from build123d import *

# Parameters (mm, degrees)
SKETCH_1_W          = 100
SKETCH_1_H          = 100
EXTRUDE_1_DEPTH     = 4
SKETCH_4_W          = 100
SKETCH_4_H          = 100
CUT_EXTRUDE_1_DEPTH = 71.823724839
SKETCH_5_R          = 5.9
EXTRUDE_2_DEPTH     = 1
SKETCH_6_R          = 1.5
SKETCH_6_R_2        = 1
CUT_EXTRUDE_2_DEPTH = 43.699531613
SKETCH_7_R          = 2.5
CUT_EXTRUDE_3_DEPTH = 2


with BuildPart() as part:
    # Эскиз1 → Бобышка-Вытянуть1 (new body)
    with BuildSketch(Plane(origin=(0, 0, 0), x_dir=(1, 0, 0), z_dir=(0, 1, 0))):
        Rectangle(SKETCH_1_W, SKETCH_1_H)
    extrude(amount=EXTRUDE_1_DEPTH)

    # Эскиз4 → Вырез-Вытянуть1 (cut, through all)
    with BuildSketch(Plane(origin=(0, 4, 0), x_dir=(1, 0, 0), z_dir=(0, 1, 0))):
        Rectangle(SKETCH_4_W, SKETCH_4_H)
        with BuildLine():
            Line((3.546261356, 21.75), (5.566987298, 25.25))
            ThreePointArc((5.566987298, 25.25), (5.566987298, 25.75), (5.133974596, 26))
            Line((5.133974596, 26), (-5.133974596, 26))
            ThreePointArc((-5.133974596, 26), (-5.566987298, 25.75), (-5.566987298, 25.25))
            Line((-5.566987298, 25.25), (-3.546261356, 21.75))
            ThreePointArc((-3.546261356, 21.75), (-3.546261356, 21.25), (-3.979274058, 21))
            Line((-3.979274058, 21), (-13, 21))
            ThreePointArc((-13, 21), (-17.862198755, 19.352875197), (-20.722235468, 15.089755817))
            ThreePointArc((-20.722235468, 15.089755817), (-23.196926567, 10.739563503), (-27.469608288, 8.133328648))
            ThreePointArc((-27.469608288, 8.133328648), (-33.5, 0), (-27.469608288, -8.133328648))
            ThreePointArc((-27.469608288, -8.133328648), (-23.196926567, -10.739563503), (-20.722235468, -15.089755817))
            ThreePointArc((-20.722235468, -15.089755817), (-17.862198755, -19.352875197), (-13, -21))
            Line((-13, -21), (13, -21))
            ThreePointArc((13, -21), (17.862198755, -19.352875197), (20.722235468, -15.089755817))
            ThreePointArc((20.722235468, -15.089755817), (23.196926567, -10.739563503), (27.469608288, -8.133328648))
            ThreePointArc((27.469608288, -8.133328648), (33.5, 0), (27.469608288, 8.133328648))
            ThreePointArc((27.469608288, 8.133328648), (23.196926567, 10.739563503), (20.722235468, 15.089755817))
            ThreePointArc((20.722235468, 15.089755817), (17.862198755, 19.352875197), (13, 21))
            Line((13, 21), (3.979274058, 21))
            ThreePointArc((3.979274058, 21), (3.546261356, 21.25), (3.546261356, 21.75))
        make_face(mode=Mode.SUBTRACT)
    extrude(amount=-CUT_EXTRUDE_1_DEPTH, mode=Mode.SUBTRACT)

    # Эскиз5 → Бобышка-Вытянуть2 (add)
    with BuildSketch(Plane.XZ):
        with Locations(Location((25, 0, 0), (0, 0, 270))):
            Circle(SKETCH_5_R)
        with Locations(Location((-25, 0, 0), (0, 0, 270))):
            Circle(SKETCH_5_R)
        with BuildLine():
            Line((-0.970460198, 14.023475383), (0.970460198, 14.023475383))
            ThreePointArc((0.970460198, 14.023475383), (1.700884179, 14.199930228), (2.270199596, 14.690374372))
            ThreePointArc((2.270199596, 14.690374372), (15.793250353, 15.793250353), (14.690374372, 2.270199596))
            ThreePointArc((14.690374372, 2.270199596), (14.199930228, 1.700884179), (14.023475383, 0.970460198))
            Line((14.023475383, 0.970460198), (14.023475383, -0.970460198))
            ThreePointArc((14.023475383, -0.970460198), (14.199930228, -1.700884179), (14.690374372, -2.270199596))
            ThreePointArc((14.690374372, -2.270199596), (15.793250353, -15.793250353), (2.270199596, -14.690374372))
            ThreePointArc((2.270199596, -14.690374372), (1.700884179, -14.199930228), (0.970460198, -14.023475383))
            Line((0.970460198, -14.023475383), (-0.970460198, -14.023475383))
            ThreePointArc((-0.970460198, -14.023475383), (-1.700884179, -14.199930228), (-2.270199596, -14.690374372))
            ThreePointArc((-2.270199596, -14.690374372), (-15.793250353, -15.793250353), (-14.690374372, -2.270199596))
            ThreePointArc((-14.690374372, -2.270199596), (-14.199930228, -1.700884179), (-14.023475383, -0.970460198))
            Line((-14.023475383, -0.970460198), (-14.023475383, 0.970460198))
            ThreePointArc((-14.023475383, 0.970460198), (-14.199930228, 1.700884179), (-14.690374372, 2.270199596))
            ThreePointArc((-14.690374372, 2.270199596), (-15.793250353, 15.793250353), (-2.270199596, 14.690374372))
            ThreePointArc((-2.270199596, 14.690374372), (-1.700884179, 14.199930228), (-0.970460198, 14.023475383))
        make_face()
    extrude(amount=EXTRUDE_2_DEPTH)

    # Эскиз6 → Вырез-Вытянуть2 (cut, through all)
    # profile 1 of 4: a face of its own
    with BuildSketch(Plane(origin=(0, 4, 0), x_dir=(1, 0, 0), z_dir=(0, 1, 0))):
        with Locations(Location((0, 17.5, 0), (0, 0, 270))):
            Circle(SKETCH_6_R)
        with Locations((0, 17.5)):
            Circle(SKETCH_6_R_2, mode=Mode.SUBTRACT)
    # profile 2 of 4: a face of its own
    with BuildSketch(Plane(origin=(0, 4, 0), x_dir=(1, 0, 0), z_dir=(0, 1, 0))):
        with Locations((0, 17.5)):
            Circle(SKETCH_6_R_2)
    # profile 3 of 4: a face of its own
    with BuildSketch(Plane(origin=(0, 4, 0), x_dir=(1, 0, 0), z_dir=(0, 1, 0))):
        with Locations(Location((0, -17.5, 0), (0, 0, 270))):
            Circle(SKETCH_6_R)
        with Locations((0, -17.5)):
            Circle(SKETCH_6_R_2, mode=Mode.SUBTRACT)
    # profile 4 of 4: a face of its own
    with BuildSketch(Plane(origin=(0, 4, 0), x_dir=(1, 0, 0), z_dir=(0, 1, 0))):
        with Locations((0, -17.5)):
            Circle(SKETCH_6_R_2)
    extrude(amount=-CUT_EXTRUDE_2_DEPTH, mode=Mode.SUBTRACT)

    # Эскиз7 → Вырез-Вытянуть3 (cut)
    with BuildSketch(Plane(origin=(0, 4, 0), x_dir=(1, 0, 0), z_dir=(0, 1, 0))):
        with Locations(Location((0, 17.5, 0), (0, 0, 270))):
            Circle(SKETCH_7_R)
        with Locations(Location((0, -17.5, 0), (0, 0, 270))):
            Circle(SKETCH_7_R)
    extrude(amount=-CUT_EXTRUDE_3_DEPTH, mode=Mode.SUBTRACT)


solid = part.part
The listing builds one solid part. Answer for the finished solid, in the listing's coordinates (mm). A direction names the side the tool comes from. Give positions to 0.01 mm unless a question says otherwise; leave off trailing zeros. Loops run counter-clockwise (first coordinate to the right, second up) from the corner with the lowest first, then second, coordinate; pieces in that order, holes last. Notation, with made-up numbers: (33, -16.5) - (69, -16.5) arc R37 cw to (69, 22.5) - close; hole circle Ø10 at (0.25, 44). An arc over 180 degrees is marked (long way). Use one line per item in the form item = value.
1. Section D-D on z = -17.5 is taken. Give the vertices of the cut face in (x, y).
Calculated:
outline = (-19.61, 0) - (-13.4, 0) - (-13.4, -1) - (-5.6, -1) - (-5.6, 0) - (-1.5, 0) - (-1.5, 2) - (-2.5, 2) - (-2.5, 4) - (-19.61, 4) - close; (1.5, 0) - (5.6, 0) - (5.6, -1) - (13.4, -1) - (13.4, 0) - (19.61, 0) - (19.61, 4) - (2.5, 4) - (2.5, 2) - (1.5, 2) - close
2. Find the intervals of material crossed by line 1 along Y through (x, z) = (23, -6); line 2 along Z through (x, y) = (-8, 1.3); line 3 along X through (y, z) = (2.5, 17.5), in increasing order. Write a range as [from, to].
Calculated:
line_1 = [0, 4]
line_2 = [-21, 21]
line_3 = [-19.61, -2.5], [2.5, 19.61]
3. Given pin 1 Ø0.8 at (x, y) = (0.5, -0.5) entering from +Z; pin 2 Ø3.5 at (x, z) = (0, -17.5) entering from -Y; pin 3 Ø1 at (x, y) = (9.5, 0) entering from -Z, each flat-ended and moving along its own axis, determine where each tip first touches the part or whether it passes through.
Calculated:
pin_1 = 14.02
pin_2 = 0
pin_3 = -21
4. The mould has two halves that part along Z. Classify faces 1 (the face through (25, -1, 0)), 2 (the face through (17.92, 2.03, -19.31)), 3 (the face through (-23.246, 2.028, 10.689)), 4 (the face through (4.542, 2.028, -23.476)): pulls with the +Z half, pulls with the -Z half, needs draft (parallel to the pull), parting line crosses it, or undercut.
Calculated:
face_1 = needs draft
face_2 = pulls with the -Z half
face_3 = pulls with the +Z half
face_4 = undercut
5. Section C-C on x = -9.5 is taken. Give the vertices of the cut face in (y, z).
Calculated:
outline = (-1, -18.4) - (0, -18.4) - (0, -21) - (4, -21) - (4, 21) - (0, 21) - (0, 18.4) - (-1, 18.4) - close
6. Which of the six approach directions +Z, -Z, +X, -X, +Y, -Y give full straight-line access (tool end or side, diameter ignored) to faces 5 (the face through (23.15, 2.03, 10.79)), 6 (the face through (-8, 2, -21)), 7 (the face through (-17.92, 2.03, 19.31)), 8 (the face through (-20.025, -0.493, -3.172)), 9 (the face through (-1, 2, 19))?
Calculated:
face_5 = +Z, +X, +Y, -Y
face_6 = -X, +Y, -Y
face_7 = +Z, -X, +Y, -Y
face_8 = -Y
face_9 = +Y
7. Section B-B on z = 0 is taken. Give the vertices of the cut face in (x, y).
Calculated:
outline = (-33.5, 0) - (-30.9, 0) - (-30.9, -1) - (-19.1, -1) - (-19.1, 0) - (-14.02, 0) - (-14.02, -1) - (14.02, -1) - (14.02, 0) - (19.1, 0) - (19.1, -1) - (30.9, -1) - (30.9, 0) - (33.5, 0) - (33.5, 4) - (-33.5, 4) - close
8. Section A-A on y = 1 is taken. Give the vertices of the cut face in (x, z), then the cut area to 3 significant figures.
Calculated:
outline = (-27.47, -8.13) arc R10 cw to (-20.72, -15.09) arc R8 ccw to (-13, -21) - (-3.98, -21) arc R0.5 cw to (-3.55, -21.75) - (-5.57, -25.25) arc R0.5 ccw to (-5.13, -26) - (5.13, -26) arc R0.5 ccw to (5.57, -25.25) - (3.55, -21.75) arc R0.5 cw to (3.98, -21) - (13, -21) arc R8 ccw to (20.72, -15.09) arc R10 cw to (27.47, -8.13) arc R8.5 ccw to (27.47, 8.13) arc R10 cw to (20.72, 15.09) arc R8 ccw to (13, 21) - (-13, 21) arc R8 ccw to (-20.72, 15.09) arc R10 cw to (-27.47, 8.13) arc R8.5 ccw to start; hole circle Ø3 at (0, -17.5); hole circle Ø3 at (0, 17.5)
area = 2,150 mm^2
